The model under review builds one solid part; all positions refer to its coordinate system, in mm. A direction names the side the tool comes from. Round coordinates to 2 decimals unless told otherwise and drop trailing zeros. Loops run counter-clockwise (first coordinate to the right, second up) from the corner with the lowest first, then second, coordinate; pieces in that order, holes last. Notation, with made-up numbers: (-14, 86.25) -> (1, 86.25) arc R24 cw to (1, 123.25) -> close; hole circle Ø1 at (-27.5, 1.25). An arc over 180 degrees is marked (long way). Use a Markdown table: item, result. Add a question column.
1) Consider section C-C on y = -12.7. Give the boundary of the cut face in (x, z) (3 decimals), plus the area to 3 significant figures.
2) Mouldability with a two-part tool opening along X and no side actions: class faces 3 (the flat face through (0, -75, 21)), 4 (the flat face through (13, 0, 2)), 5 (the cylindrical face through (10.18, -10.77, 1.57)) as released by +X, released by -X, zero draft, split by the parting line, or undercut.
3) Consider section B-B on x = 12.7. Give the boundary of the cut face in (y, z) (3 decimals).
4) Consider section D-D on x = 2. Give the boundary of the cut face in (y, z) (3 decimals), plus the area to 3 significant figures.
5) For faces 1 (the flat face through (25.4, -55, 1)), 2 (the flat face through (10, -36, 3.175)), list the 3-axis set-ups (+Z, -Z, +X, -X, +Y, -Y) from which the entire face can be reached by the end or side of a thin tool; tool diameter is ignored.
6) Insertion check: pin 1 (5.5 mm diameter, centred on x = 12.7, y = -38.1, fed in from +Z); pin 2 (2 mm diameter, centred on x = 7.5, y = -36, fed in from +Z) (3 decimals); pin 3 (4 mm diameter, centred on x = 18, z = 21.5, fed in from +Y) (3 decimals). Each pin has a flat end and moves straight along its axis. Give the tip position at first contact, or say it passes through.
7) Consider section A-A on z = 63.5. Give the boundary of the cut face in (x, y) (3 decimals).
8) Wall thickness on probe 1 along Y at (x, z) = (12.7, 2.1) (3 decimals); probe 2 along Z at (x, y) = (12.7, -74.7) (3 decimals); probe 3 along X at (y, z) = (-75.4, 63.5) (3 decimals): over which ranges is each line inside the solid? List them lowest first.
Autodesk Inventor part; units mm, degrees
ref_plane "YZ Plane" through (0, 0, 0) normal (1, 0, 0) x (0, 1, 0)
ref_plane "XZ Plane" through (0, 0, 0) normal (0, 1, 0) x (-1, 0, 0)
ref_plane "XY Plane" through (0, 0, 0) normal (0, 0, 1) x (1, 0, 0)
sketch "Sketch1" plane through (0, 0, 0) normal (0, 0, 1) x (1, 0, 0)
  line L0 (0, 0) -> (25.4, 0)
  line L1 (25.4, 0) -> (25.4, -76.2)
  line L2 (25.4, -76.2) -> (0, -76.2)
  line L3 (0, -76.2) -> (0, 0)
  circle A0 centre (12.7, -12.7) radius 3.175
  circle A1 centre (12.7, -38.1) radius 3.175
  dimension "d0" = 25.4
  dimension "d1" = 76.2
  dimension "d2" = 6.35
  dimension "d3" = 6.35
  dimension "d4" = 12.7
  dimension "d5" = 12.7
  dimension "d6" = 12.7
  dimension "d7" = 25.4
extrude "Extrusion1" add sketch "Sketch1" along normal blind 3.175
sketch "Sketch2" plane through (0, 0, 3.175) normal (0, 0, 1) x (1, 0, 0)
  line L0 (25.4, -76.2) -> (25.4, 0)
  line L1 (0, 0) -> (0, -76.2)
  line L2 (25.4, -76.2) -> (0, -76.2)
  line L3 (0, -76.2) -> (0, -73.025)
  line L4 (0, -73.025) -> (25.4, -73.025)
  line L5 (25.4, -73.025) -> (25.4, -76.2)
  dimension "d10" = 3.175
extrude "Extrusion2" add sketch "Sketch2" along normal blind 73.025
sketch "Sketch3" plane through (0, -73.025, 3.175) normal (0, 1, 0) x (1, 0, 0)
  circle A0 centre (12.7, -60.325) radius 3.175
  circle A1 centre (12.7, -34.925) radius 3.175
  line L0 (0, 0) -> (0, -73.025)
  line L1 (25.4, -73.025) -> (0, -73.025)
  point P0 (0, 3.175)
  dimension "d13" = 6.35
  dimension "d14" = 6.35
  dimension "d15" = 12.7
  dimension "d16" = 12.7
  dimension "d17" = 12.7
  dimension "d18" = 25.4
extrude "Extrusion3" cut sketch "Sketch3" against normal blind 73.025
properties part number "15102898-16-P-0510" material "Stainless Steel"
Result set:
| question | item | result |
|---|---|---|
| 1 | outline | (0, 0) -> (9.525, 0) -> (9.525, 3.175) -> (0, 3.175) -> close; (15.875, 0) -> (25.4, 0) -> (25.4, 3.175) -> (15.875, 3.175) -> close |
| 1 | area | 60.5 mm2 |
| 2 | face 3 | released by -X |
| 2 | face 4 | zero draft |
| 2 | face 5 | undercut |
| 3 | outline | (-76.2, 0) -> (-41.275, 0) -> (-41.275, 3.175) -> (-73.025, 3.175) -> (-73.025, 34.925) -> (-76.2, 34.925) -> close; (-76.2, 41.275) -> (-73.025, 41.275) -> (-73.025, 60.325) -> (-76.2, 60.325) -> close; (-76.2, 66.675) -> (-73.025, 66.675) -> (-73.025, 76.2) -> (-76.2, 76.2) -> close; (-34.925, 0) -> (-15.875, 0) -> (-15.875, 3.175) -> (-34.925, 3.175) -> close; (-9.525, 0) -> (0, 0) -> (0, 3.175) -> (-9.525, 3.175) -> close |
| 4 | outline | (-76.2, 0) -> (0, 0) -> (0, 3.175) -> (-73.025, 3.175) -> (-73.025, 76.2) -> (-76.2, 76.2) -> close |
| 4 | area | 474 mm2 |
| 5 | face 1 | +Z, -Z, +X, +Y, -Y |
| 5 | face 2 | +Z, +X, -X, +Y |
| 6 | pin 1 | through |
| 6 | pin 2 | z = 3.175 |
| 6 | pin 3 | y = -73.025 |
| 7 | outline | (0, -76.2) -> (9.525, -76.2) -> (9.525, -73.025) -> (0, -73.025) -> close; (15.875, -76.2) -> (25.4, -76.2) -> (25.4, -73.025) -> (15.875, -73.025) -> close |
| 8 | probe 1 | -76.2 to -41.275, -34.925 to -15.875, -9.525 to 0 |
| 8 | probe 2 | 0 to 34.925, 41.275 to 60.325, 66.675 to 76.2 |
| 8 | probe 3 | 0 to 9.525, 15.875 to 25.4 |
